Build history of the part. All positions in model axes, mm. A direction names the side the tool comes from. Give positions to 0.01 mm unless a question says otherwise; leave off trailing zeros. Loops run counter-clockwise (first coordinate to the right, second up) from the corner with the lowest first, then second, coordinate; pieces in that order, holes last. Notation, with made-up numbers: (-13, 74) -> (13, 74) arc R25 cw to (13, 99) -> close; hole circle Ø4 at (77.5, 78). An arc over 180 degrees is marked (long way). Answer as a JSON object with one key per item and string values. Group by question number.
Q1. Band-saw the part on A-A, the plane y = -28. Write the cut outline in (x, z) (3 decimals), plus the area to 3 significant figures.
Q2. Two-plate mould, pull along X, no slides. Class faces 3 (the cylindrical face through (-74.751, -38.562, 74.672)), 4 (the flat face through (-16, -25.4, 55)), 5 (the cylindrical face through (-1.449, -38.562, 74.672)), 6 (the cylindrical face through (-37.638, -1.528, 74.751)): pulls with the +X half, pulls with the -X half, needs draft (parallel to the pull), parting line crosses it, or undercut.
Q3. Wall check: probe 1 along X at (y, z) = (-71, 60.5) (3 decimals); probe 2 along Z at (x, y) = (-53, -51.5); probe 3 along Z at (x, y) = (-15, -70.5). Give the ranges that are in metal, low to high. Write a range as from..to.
Q4. Drop a flat-ended pin along its axis: pin 1 (6.5 mm diameter, centred on x = -60.5, z = 53, fed in from -Y). Give the stop position or say it passes through.
Q5. Tool access for faces 1 (the flat face through (-39, -38, 0)), 2 (the flat face through (-41, -51, 30.702)): list every direction of +Z, -Z, +X, -X, +Y, -Y with a clear straight run to the whole face (end or side of a thin tool).
Q6. Band-saw the part on B-B, the plane z = 58. Write the cut outline in (x, y) (3 decimals), plus the area to 3 significant figures.
Q7. Band-saw the part on C-C, the plane x = -31. Write the cut outline in (y, z).
from build123d import *

# Parameters (mm, degrees)
F0_W     = 76.2
F0_H     = 76.2
F1_DEPTH = 76.2
F3_R     = 5.08
F2_W     = 12.7
F2_H     = 12.7
F2_W_2   = 25.4
F4_DEPTH = 50.8


with BuildPart() as f1:
    # F0 (on Front) → F1 (new body)
    with BuildSketch(Plane.XZ):
        with Locations((-38.1, 38.1)):
            Rectangle(F0_W, F0_H)
    extrude(amount=F1_DEPTH)

    # F3
    f3_edges = [f1.edges().sort_by_distance(p)[0] for p in [
        (-38.1, -76.2, 0),
        (0, -76.2, 38.1),
        (-38.1, -76.2, 76.2),
        (-76.2, -76.2, 38.1),
        (0, -38.1, 0),
        (0, -38.1, 76.2),
        (0, 0, 38.1),
        (-76.2, -38.1, 76.2),
        (-76.2, -38.1, 0),
        (-76.2, 0, 38.1),
        (-38.1, 0, 0),
        (-38.1, 0, 76.2),
    ]]
    fillet(f3_edges, radius=F3_R)

    # F2 (on face) → F4 (cut)
    with BuildSketch(Plane.XZ.offset(76.2)):
        with Locations((-60.229752, 54.895747)):
            Rectangle(F2_W, F2_H)
        with Locations((-15.875, 54.578253)):
            Rectangle(F2_W, F2_H)
        with Locations((-41.306752, 24.352249)):
            Rectangle(F2_W_2, F2_H)
    extrude(amount=-F4_DEPTH, mode=Mode.SUBTRACT)


solid = f1.part
Worked answers:
{
 "1": {"outline": "(-76.2, 5.08) arc R5.08 ccw to (-71.12, 0) -> (-5.08, 0) arc R5.08 ccw to (0, 5.08) -> (0, 71.12) arc R5.08 ccw to (-5.08, 76.2) -> (-71.12, 76.2) arc R5.08 ccw to (-76.2, 71.12) -> close; hole (-66.58, 48.546) -> (-53.88, 48.546) -> (-53.88, 61.246) -> (-66.58, 61.246) -> close; hole (-54.007, 18.002) -> (-28.607, 18.002) -> (-28.607, 30.702) -> (-54.007, 30.702) -> close; hole (-22.225, 48.228) -> (-9.525, 48.228) -> (-9.525, 60.928) -> (-22.225, 60.928) -> close", "area": "5,140 mm2"},
 "2": {"face 3": "pulls with the -X half", "face 4": "undercut", "face 5": "pulls with the +X half", "face 6": "needs draft"},
 "3": {"probe 1": "-76.2..-66.58, -53.88..-22.225, -9.525..0", "probe 2": "0..18, 30.7..76.2", "probe 3": "0..48.23, 60.93..76.2"},
 "4": {"pin 1": "y = -25.4"},
 "5": {"face 1": "-Z, +X, -X, +Y, -Y", "face 2": "-Y"},
 "6": {"outline": "(-76.2, -71.12) arc R5.08 ccw to (-71.12, -76.2) -> (-66.58, -76.2) -> (-66.58, -25.4) -> (-53.88, -25.4) -> (-53.88, -76.2) -> (-22.225, -76.2) -> (-22.225, -25.4) -> (-9.525, -25.4) -> (-9.525, -76.2) -> (-5.08, -76.2) arc R5.08 ccw to (0, -71.12) -> (0, -5.08) arc R5.08 ccw to (-5.08, 0) -> (-71.12, 0) arc R5.08 ccw to (-76.2, -5.08) -> close", "area": "4,490 mm2"},
 "7": {"outline": "(-76.2, 5.08) arc R5.08 ccw to (-71.12, 0) -> (-5.08, 0) arc R5.08 ccw to (0, 5.08) -> (0, 71.12) arc R5.08 ccw to (-5.08, 76.2) -> (-71.12, 76.2) arc R5.08 ccw to (-76.2, 71.12) -> (-76.2, 30.7) -> (-25.4, 30.7) -> (-25.4, 18) -> (-76.2, 18) -> close"}
}
